```python
from build123d import *

# Parameters (mm, degrees)
MAINBLOCK_DEPTH               = 3.81
BOSS_EXTRUDE1_DEPTH           = 16.51
SKETCH3_R                     = 1.6256
CUT_EXTRUDE1_DEPTH            = 131.252044518
FILLET1_R                     = 1.27
SKETCH4_W                     = 30.48
SKETCH4_H                     = 2.54
STABILIZER_MOUNT_CUTOUT_DEPTH = 9.271
FILLET2_R                     = 1.905


with BuildPart() as part:
    # Sketch1 → MainBlock (new body)
    with BuildSketch(Plane(origin=(0, 0, 0), x_dir=(1, 0, 0), z_dir=(0, 1, 0))):
        with BuildLine():
            Line((-99.441, 24.384), (99.441, 24.384))
            ThreePointArc((99.441, 24.384), (123.825, 0), (99.441, -24.384))
            Line((99.441, -24.384), (-99.441, -24.384))
            ThreePointArc((-99.441, -24.384), (-123.825, 0), (-99.441, 24.384))
        make_face()
    extrude(amount=MAINBLOCK_DEPTH)

    # Sketch2 → Boss-Extrude1 (add)
    with BuildSketch(Plane.XZ):
        with BuildLine():
            Line((-99.441, 26.924), (99.441, 26.924))
            ThreePointArc((99.441, 26.924), (126.365, 0), (99.441, -26.924))
            Line((99.441, -26.924), (-99.441, -26.924))
            ThreePointArc((-99.441, -26.924), (-126.365, 0), (-99.441, 26.924))
        make_face()
        with BuildLine():
            Line((99.441, 24.384), (-99.441, 24.384))
            ThreePointArc((-99.441, 24.384), (-123.825, 0), (-99.441, -24.384))
            Line((-99.441, -24.384), (99.441, -24.384))
            ThreePointArc((99.441, -24.384), (123.825, 0), (99.441, 24.384))
        make_face(mode=Mode.SUBTRACT)
    extrude(amount=-BOSS_EXTRUDE1_DEPTH)

    # Sketch3 → Cut-Extrude1 (cut, through all)
    with BuildSketch(Plane.XZ):
        with Locations(Location((-68.961, 0, 0), (0, 0, 270))):
            Circle(SKETCH3_R)
        with Locations(Location((68.961, 0, 0), (0, 0, 270))):
            Circle(SKETCH3_R)
    extrude(amount=-CUT_EXTRUDE1_DEPTH, mode=Mode.SUBTRACT)

    # Fillet1
    fillet1_edges = [part.edges().sort_by_distance(p)[0] for p in [
        (123.825, 3.81, 0),
        (0, 3.81, -24.384),
        (-123.825, 3.81, 0),
        (0, 3.81, 24.384),
    ]]
    fillet(fillet1_edges, radius=FILLET1_R)

    # Sketch4 → Stabilizer-Mount-Cutout (cut)
    with BuildSketch(Plane(origin=(0, 16.51, 0), x_dir=(1, 0, 0), z_dir=(0, 1, 0))):
        with Locations((15.621, 25.654)):
            Rectangle(SKETCH4_W, SKETCH4_H)
    stabilizer_mount_cutout = extrude(amount=-STABILIZER_MOUNT_CUTOUT_DEPTH, mode=Mode.SUBTRACT)

    # Mirror1: Stabilizer-Mount-Cutout across plane
    add(stabilizer_mount_cutout.mirror(Plane.XY), mode=Mode.SUBTRACT)

    # Fillet2
    fillet2_edges = [part.edges().sort_by_distance(p)[0] for p in [
        (30.861, 7.239, -25.654),
        (0.381, 7.239, -25.654),
        (0.381, 7.239, 25.654),
        (30.861, 7.239, 25.654),
    ]]
    fillet(fillet2_edges, radius=FILLET2_R)


solid = part.part
```
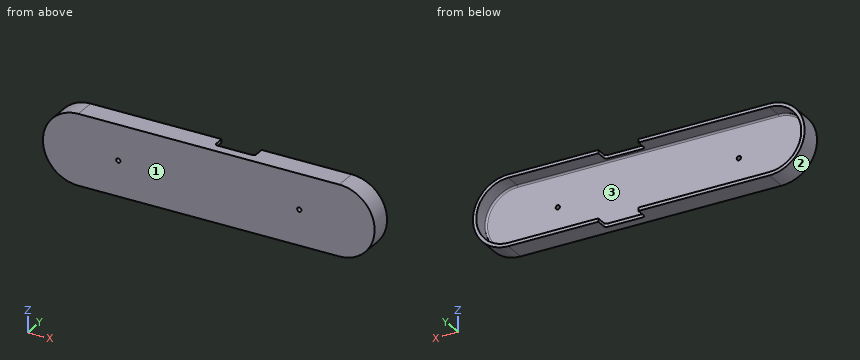
Geometry: final body of the model. Coordinates: model frame, mm. Face numbers are marked on the shaded views. Round coordinates to 2 decimals unless told otherwise and drop trailing zeros. Order: outer loops, then holes, each group sorted by start corner. A loop starts at its lowest first (then second) coordinate and runs counter-clockwise, first axis right, second up. Notation, with made-up numbers: M 21.5,67 L 29.5,67 A16 ccw 29.5,75 Z; hole C 10,76.25 d6. An arc over 180 degrees is marked long. Use one line per item in the form item = value. Start each with the question number.
Q1. Cut plane A-A (x = 36). Return loops of the section in (y, z), and give its area (3 significant figures).
Q2. Mould query, pull axis Z, two halves, no side actions, for the marked faces 1, 2 and 3. Classes: +Z half, -Z half, draft (parallel to the pull), parting line (faces both ways), or undercut.
Q3. Material intervals for line 1 (X direction, y = 2.9, z = 0) (3 decimals); line 2 (Z direction, x = -25.5, y = 5.5); line 3 (X direction, y = 9.5, z = -1.5), sorted ascending. Write a range as [from, to].
Q4. Pin query (flat end, axial travel): pin 1 Ø6 at (x, z) = (17.5, 12) entering from +Y; pin 2 Ø0.8 at (y, z) = (12.5, 25) entering from -X; pin 3 Ø8 at (y, z) = (11, 11.5) entering from +X. Return the tip coordinate at first contact, or that it passes through.
Q5. Cut plane B-B (x = 7). Return loops of the section in (y, z).
Geometry results:
q1.outline = M 0,-26.92 L 16.51,-26.92 L 16.51,-24.38 L 5.08,-24.38 A1.27 cw 3.81,-23.11 L 3.81,23.11 A1.27 cw 5.08,24.38 L 16.51,24.38 L 16.51,26.92 L 0,26.92 Z
q1.area = 270 mm^2
q2.face_1 = draft
q2.face_2 = parting line
q2.face_3 = undercut
q3.line_1 = [-126.365, -70.587], [-67.335, 67.335], [70.587, 126.365]
q3.line_2 = [-26.92, -24.38], [24.38, 26.92]
q3.line_3 = [-126.32, -123.78], [123.78, 126.32]
q4.pin_1 = 3.81
q4.pin_2 = -110.38
q4.pin_3 = 125.3
q5.outline = M 0,-26.92 L 7.24,-26.92 L 7.24,-24.38 L 5.08,-24.38 A1.27 cw 3.81,-23.11 L 3.81,23.11 A1.27 cw 5.08,24.38 L 7.24,24.38 L 7.24,26.92 L 0,26.92 Z
